Read the model definition and answer for the solid it produces. Units are mm, in the model's axes. A direction names the side the tool comes from. Give positions to 0.01 mm unless a question says otherwise; leave off trailing zeros. Order: outer loops, then holes, each group sorted by start corner. A loop starts at its lowest first (then second) coordinate and runs counter-clockwise, first axis right, second up. Notation, with made-up numbers: (37, 66.25) - (60, 66.25) arc R24 cw to (60, 102.25) - close; hole circle Ø4 at (83.5, 49.5). An arc over 180 degrees is marked (long way). Write each question's results on one line, items separated by ' | '. Start each with the question number.
Q1. For a pull along Y with two mould halves and no side action, classify faces 1 (the face through (-22.459, 55, -24)), 2 (the face through (-24, 7.541, -24)), 3 (the face through (-32, -5.441, -24)) as +Y half, -Y half, draft (parallel to the pull), parting line (faces both ways), or undercut.
Q2. Find the intervals of material crossed by line 1 along Y through (x, z) = (-47.5, -23.2); line 2 along Y through (x, z) = (-37.5, -24.8); line 3 along X through (y, z) = (44.5, -23.5), in increasing order. Write a range as from..to.
Q3. Find section B-B on x = -47.5. Give the vertices of the cut face in (y, z) (3 decimals), and give its area (3 significant figures).
Q4. Find section C-C on y = 25.5. Give the vertices of the cut face in (x, z) (3 decimals).
Q5. Find section D-D on z = -23.7. Count the separate pieces of the cut face and the enclosed holes in it, and give its area (3 significant figures).
Q6. A tool of negligible diameter and unlimited length cuts with its end or side. For faces 4 (the face through (-24, 47.541, -24)), 5 (the face through (-24, 57.541, -24)), 6 (the face through (-33.166, -3, -24)), from which of +Z, -Z, +X, -X, +Y, -Y can it reach the whole face along a straight path? Write none if from no direction.
Q7. Find section A-A on y = 45. Give the vertices of the cut face in (x, z) (3 decimals).
Q8. Flat-ended cylindrical pins translate along their axes: P1, Ø1, axis at y = -3.5, z = -23.5, coming from the +X side; P2, Ø1.6, axis at x = -24.5, z = -24, coming from the +Y side; P3, Ø1, axis at y = 40.5, z = -24, coming from the +X side. Find the tip coordinate at first contact, or state that the pin passes through.
from build123d import *

# Parameters (mm, degrees)
SKETCH1_W           = 24.825
SKETCH1_H           = 3.175
SKETCH1_W_2         = 3.175
SKETCH1_H_2         = 24.825
BOSS_EXTRUDE1_DEPTH = 60
SKETCH2_W           = 3.125
SKETCH2_H           = 5.4
BOSS_EXTRUDE4_DEPTH = 3.175
SKETCH4_R           = 8
CUT_EXTRUDE1_DEPTH  = 3.175
SKETCH3_R           = 8
CUT_EXTRUDE2_DEPTH  = 3.175
SKETCH5_W           = 3.175
SKETCH5_H           = 5.4
BOSS_EXTRUDE5_DEPTH = 3.175
SKETCH6_R           = 1.75
CUT_EXTRUDE3_DEPTH  = 10
SKETCH7_R           = 1.75
CUT_EXTRUDE4_DEPTH  = 10
SKETCH8_W           = 3.175
SKETCH8_H           = 65.4
CUT_EXTRUDE6_DEPTH  = 24.825
SKETCH9_W           = 3.175
SKETCH9_H           = 2.5
SKETCH9_H_2         = 5
CUT_EXTRUDE8_DEPTH  = 10
SKETCH10_R          = 1.70936
SKETCH10_R_2        = 7.95936
BOSS_EXTRUDE6_DEPTH = 3.175


with BuildPart() as part:
    # Sketch1 → Boss-Extrude1 (new body)
    with BuildSketch(Plane(origin=(0, 0, 0), x_dir=(1, 0, 0), z_dir=(0, 1, 0))):
        with Locations((-38.0875, 24.0875)):
            Rectangle(SKETCH1_W, SKETCH1_H)
        with Locations((-24.0875, 24.0875)):
            Rectangle(SKETCH1_W_2, SKETCH1_H)
        with Locations((-24.0875, 38.0875)):
            Rectangle(SKETCH1_W_2, SKETCH1_H_2)
    extrude(amount=BOSS_EXTRUDE1_DEPTH)

    # Sketch2 → Boss-Extrude4 (add)
    with BuildSketch(Plane.XY.offset(-22.5)):
        with Locations((-42.1875, -2.7)):
            Rectangle(SKETCH2_W, SKETCH2_H)
        with Locations((-31.5625, -2.7)):
            Rectangle(SKETCH2_W, SKETCH2_H)
    extrude(amount=-BOSS_EXTRUDE4_DEPTH)

    # Sketch4 → Cut-Extrude1 (cut)
    with BuildSketch(Plane.XY.offset(-22.5)):
        with Locations((-37.5, 30)):
            Circle(SKETCH4_R)
    extrude(amount=-CUT_EXTRUDE1_DEPTH, mode=Mode.SUBTRACT)

    # Sketch3 → Cut-Extrude2 (cut)
    with BuildSketch(Plane(origin=(-22.5, 0, 0), x_dir=(0, 0, -1), z_dir=(1, 0, 0))):
        with Locations((37.5, 30)):
            Circle(SKETCH3_R)
    extrude(amount=-CUT_EXTRUDE2_DEPTH, mode=Mode.SUBTRACT)

    # Sketch5 → Boss-Extrude5 (add)
    with BuildSketch(Plane(origin=(-22.5, 0, 0), x_dir=(0, 0, -1), z_dir=(1, 0, 0))):
        with Locations((42.2625, -2.7)):
            Rectangle(SKETCH5_W, SKETCH5_H)
        with Locations((31.5875, -2.7)):
            Rectangle(SKETCH5_W, SKETCH5_H)
    extrude(amount=-BOSS_EXTRUDE5_DEPTH)

    # Sketch6 → Cut-Extrude3 (cut)
    with BuildSketch(Plane.XY.offset(-22.5)):
        with Locations((-47.5, 45)):
            Circle(SKETCH6_R)
        with Locations((-27.5, 45)):
            Circle(SKETCH6_R)
    extrude(amount=-CUT_EXTRUDE3_DEPTH, mode=Mode.SUBTRACT)

    # Sketch7 → Cut-Extrude4 (cut)
    with BuildSketch(Plane(origin=(-22.5, 0, 0), x_dir=(0, 0, -1), z_dir=(1, 0, 0))):
        with Locations((47.5, 45)):
            Circle(SKETCH7_R)
        with Locations((27.5, 45)):
            Circle(SKETCH7_R)
    extrude(amount=-CUT_EXTRUDE4_DEPTH, mode=Mode.SUBTRACT)

    # Sketch8 → Cut-Extrude6 (cut)
    with BuildSketch(Plane(origin=(0, 0, -50.5), x_dir=(-1, 0, 0), z_dir=(0, 0, -1))):
        with Locations((24.0875, 27.3)):
            Rectangle(SKETCH8_W, SKETCH8_H)
    extrude(amount=-CUT_EXTRUDE6_DEPTH, mode=Mode.SUBTRACT)

    # Sketch9 → Cut-Extrude8 (cut)
    with BuildSketch(Plane(origin=(0, 0, -25.675), x_dir=(-1, 0, 0), z_dir=(0, 0, -1))):
        with Locations((24.0875, 58.75)):
            Rectangle(SKETCH9_W, SKETCH9_H)
        with Locations((24.0875, 50)):
            Rectangle(SKETCH9_W, SKETCH9_H_2)
        with Locations((24.0875, 40)):
            Rectangle(SKETCH9_W, SKETCH9_H_2)
        with Locations((24.0875, 30)):
            Rectangle(SKETCH9_W, SKETCH9_H_2)
        with Locations((24.0875, 20)):
            Rectangle(SKETCH9_W, SKETCH9_H_2)
        with Locations((24.0875, 10)):
            Rectangle(SKETCH9_W, SKETCH9_H_2)
        with Locations((24.0875, 1.25)):
            Rectangle(SKETCH9_W, SKETCH9_H)
    extrude(amount=-CUT_EXTRUDE8_DEPTH, mode=Mode.SUBTRACT)

    # Sketch10 → Boss-Extrude6 (add)
    with BuildSketch(Plane(origin=(0, 0, -25.675), x_dir=(-1, 0, 0), z_dir=(0, 0, -1))):
        Polygon((25.63436, 60.04064), (25.63436, 57.54064), (22.45936, 57.54064), (22.45936, 52.45936), (25.63436, 52.45936), (25.63436, 47.54064), (22.45936, 47.54064), (22.45936, 42.45936), (25.63436, 42.45936), (25.63436, 37.54064), (22.45936, 37.54064), (22.45936, 32.45936), (25.63436, 32.45936), (25.63436, 27.54064), (22.45936, 27.54064), (22.45936, 22.45936), (25.63436, 22.45936), (25.63436, 17.54064), (22.45936, 17.54064), (22.45936, 12.45936), (25.63436, 12.45936), (25.63436, 7.54064), (22.45936, 7.54064), (22.45936, 2.45936), (25.63436, 2.45936), (25.63436, -0.04064), (29.95936, -0.04064), (29.95936, -5.44064), (33.16564, -5.44064), (33.16564, -0.04064), (40.58436, -0.04064), (40.58436, -5.44064), (43.79064, -5.44064), (43.79064, -0.04064), (50.54064, -0.04064), (50.54064, 60.04064), align=None)
        with Locations((27.5, 45)):
            Circle(SKETCH10_R, mode=Mode.SUBTRACT)
        with Locations((47.5, 45)):
            Circle(SKETCH10_R, mode=Mode.SUBTRACT)
        with Locations((37.5, 30)):
            Circle(SKETCH10_R_2, mode=Mode.SUBTRACT)
    extrude(amount=-BOSS_EXTRUDE6_DEPTH)


solid = part.part
Working result:
1) face 1: draft | face 2: undercut | face 3: -Y half
2) line 1: -0.04..43.29, 46.71..60.04 | line 2: -0.04..22.04, 37.96..60.04 | line 3: -50.54..-49.13, -45.87..-29.13, -25.87..-22.46
3) outline: (-0.041, -25.675) - (43.291, -25.675) - (43.291, -22.5) - (-0.041, -22.5) - close; (46.709, -25.675) - (60.041, -25.675) - (60.041, -22.5) - (46.709, -22.5) - close | area: 180 mm²
4) outline: (-50.541, -25.675) - (-44.065, -25.675) - (-44.065, -22.5) - (-50.541, -22.5) - close; (-30.935, -25.675) - (-22.459, -25.675) - (-22.459, -22.5) - (-30.935, -22.5) - close
5) separate pieces: 1 | enclosed holes: 3 | area: 1,410 mm²
6) face 4: +Z, -Z, +X | face 5: +Z, -Z, +X, +Y | face 6: +Z, -Z, -Y
7) outline: (-50.541, -25.675) - (-49.209, -25.675) - (-49.209, -22.5) - (-50.541, -22.5) - close; (-45.791, -25.675) - (-29.209, -25.675) - (-29.209, -22.5) - (-45.791, -22.5) - close; (-25.791, -25.675) - (-22.459, -25.675) - (-22.459, -22.5) - (-25.791, -22.5) - close
8) P1: x = -29.96 | P2: y = 57.54 | P3: x = -25.63
